Here's the drawing with two shaded views (mm, measured from the low corner). I have some questions. Coordinates: 2 decimals unless noted, no trailing zeros. Write each loop counter-clockwise with the first axis right and the second up, starting at its lowest first coordinate (ties: lowest second). Pieces come first, ordered by that corner, then holes.
Item 1: For P1, Ø10, axis at x = 149, y = 14.5, coming from the -Z side; P2, Ø5, axis at x = 90.5, z = 13.5, coming from the -Y side; P3, Ø5, axis at x = 167, y = 10, coming from the +Z side, each with a flat end and sliding along its axis, tell me the tip position at first contact or that it passes through.
Item 2: I want a section at A-A on x = 177.5. Please give me the cut outline in (y, z), then the cut area to 3 significant figures.
Item 3: If I drill on probe 1 along Y at (x, z) = (282.43, 2.4); probe 2 along Z at (x, y) = (6.05, 17.7); probe 3 along Z at (x, y) = (273, 7), over which ranges is the centre line in solid material (lowest first)?
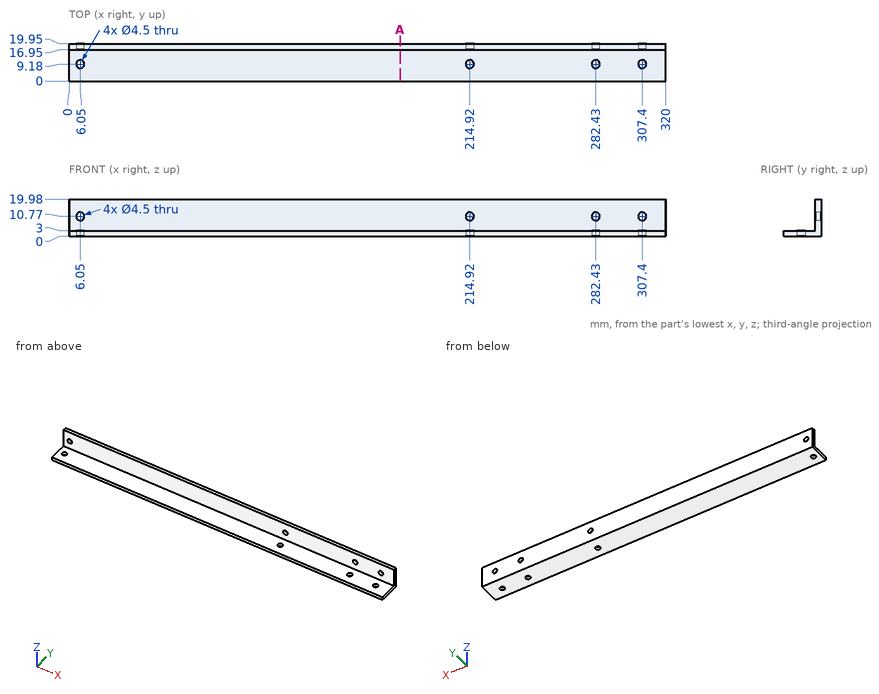
Response values:
1. P1: stops at z = 0
1. P2: stops at y = 16.95
1. P3: stops at z = 3
2. outline: (0, 0) - (19.95, 0) - (19.95, 19.98) - (16.95, 19.98) - (16.95, 3) - (0, 3) - close
2. area: 111 mm2
3. probe 1: y = 0 to 6.93, 11.43 to 19.95
3. probe 2: z = 0 to 8.52, 13.02 to 19.98
3. probe 3: z = 0 to 3
